```python
from build123d import *

# Parameters (mm, degrees)
SKETCH1_W           = 10.3
SKETCH1_H           = 5
BOSS_EXTRUDE1_DEPTH = 2.85
SKETCH2_W           = 5.7
SKETCH2_H           = 0.3
BOSS_EXTRUDE2_DEPTH = 5
SKETCH3_R           = 1.35
CUT_EXTRUDE1_DEPTH  = 5
SKETCH4_W           = 3
SKETCH4_H           = 3
BOSS_EXTRUDE3_DEPTH = 5
BOSS_EXTRUDE4_DEPTH = 0.15
LPATTERN1_COUNT     = 3
LPATTERN1_PITCH     = 3


with BuildPart() as part:
    # Sketch1 → Boss-Extrude1 (new body, symmetric)
    with BuildSketch(Plane.XY):
        Rectangle(SKETCH1_W, SKETCH1_H)
    extrude(amount=BOSS_EXTRUDE1_DEPTH, both=True)

    # Sketch2 → Boss-Extrude2 (add)
    with BuildSketch(Plane(origin=(5.15, 0, 0), x_dir=(0, 0, -1), z_dir=(1, 0, 0))):
        with Locations((0, 2.35)):
            Rectangle(SKETCH2_W, SKETCH2_H)
    boss_extrude2 = extrude(amount=BOSS_EXTRUDE2_DEPTH)

    # Sketch3 → Cut-Extrude1 (cut)
    with BuildSketch(Plane(origin=(0, 2.5, 0), x_dir=(1, 0, 0), z_dir=(0, 1, 0))):
        with Locations((7.65, 0)):
            Circle(SKETCH3_R)
    cut_extrude1 = extrude(amount=-CUT_EXTRUDE1_DEPTH, mode=Mode.SUBTRACT)

    # Mirror1: Boss-Extrude2, Cut-Extrude1 across plane
    add(boss_extrude2.mirror(Plane(origin=(0, 0, 0), x_dir=(0, 0, 1), z_dir=(1, 0, 0))))
    add(cut_extrude1.mirror(Plane(origin=(0, 0, 0), x_dir=(0, 0, 1), z_dir=(1, 0, 0))), mode=Mode.SUBTRACT)

    # Sketch4 → Boss-Extrude3 (add)
    with BuildSketch(Plane(origin=(0, 2.5, 0), x_dir=(1, 0, 0), z_dir=(0, 1, 0))):
        with Locations((2.65, 0)):
            Rectangle(SKETCH4_W, SKETCH4_H)
    extrude(amount=BOSS_EXTRUDE3_DEPTH)

    # Sketch5 → Boss-Extrude4 (add, symmetric)
    with BuildSketch(Plane.XY):
        with BuildLine():
            Line((-3.65, -2.5), (-2.15, -2.5))
            Line((-2.15, -2.5), (-2.15, -4.75))
            ThreePointArc((-2.15, -4.75), (-2.9, -5.5), (-3.65, -4.75))
            Line((-3.65, -4.75), (-3.65, -2.5))
        make_face()
        with BuildLine():
            Line((-2.45, -4.15), (-2.45, -4.75))
            ThreePointArc((-2.45, -4.75), (-2.9, -5.2), (-3.35, -4.75))
            Line((-3.35, -4.75), (-3.35, -4.15))
            ThreePointArc((-3.35, -4.15), (-2.9, -3.7), (-2.45, -4.15))
        make_face(mode=Mode.SUBTRACT)
    boss_extrude4 = extrude(amount=BOSS_EXTRUDE4_DEPTH, both=True)

    # LPattern1: Boss-Extrude4 ×3
    with Locations(*[(i * LPATTERN1_PITCH, 0, 0) for i in range(1, LPATTERN1_COUNT)]):
        add(boss_extrude4)


solid = part.part
```
Model file for the job. Use its own axes, mm. A direction names the side the tool comes from. Give positions to 0.01 mm unless a question says otherwise; leave off trailing zeros. Write each loop counter-clockwise with the first axis right and the second up, starting at its lowest first coordinate (ties: lowest second). Pieces come first, ordered by that corner, then holes. Notation, with made-up numbers: (-10.75, 83.25) -> (17.25, 83.25) arc R24 cw to (17.25, 121.25) -> close; hole circle Ø4 at (63.25, -12.5). An arc over 180 degrees is marked (long way). Use CSV: the item, a comma, the result in double quotes. Start each with the question number.
1) Pin check, flat tips, straight feed: P1, Ø3, axis at x = 7.65, z = 0, coming from the +Y side; P2, Ø0.8, axis at x = -2.5, y = -4, coming from the -Z side; P3, Ø1.5, axis at y = -4, z = -0.5, coming from the +X side. Stop position of each tip, or through.
2) Tool access for faces 1 (the flat face through (-3.2, -3.6, 0.15)), 2 (the flat face through (1.15, 5, 0)), 3 (the flat face through (2.8, -3.6, -0.15)), 4 (the flat face through (5.15, 0, 0)), 5 (the flat face through (-6, 2.2, 0)): list every direction of +Z, -Z, +X, -X, +Y, -Y with a clear straight run to the whole face (end or side of a thin tool).
3) Drill centre lines: L1, parallel to X at y = 2.45, z = 0; L2, parallel to Z at x = -7.65, y = 2.3; L3, parallel to Y at x = 1.25, z = -1.3. Where is each one in solid material? Low to high.
4) Cut at B-B on z = -1.75. List the corners of the cut face in (x, y), plus the area to 3 significant figures.
5) Cut at D-D on y = 4. List the corners of the cut face in (x, z), plus the area to 3 significant figures.
6) Cut at A-A on x = 3.1. List the corners of the cut face in (y, z).
7) Cut at C-C on x = -7.65. List the corners of the cut face in (y, z).
8) Two-plate mould, pull along X, no slides. Class faces 6 (the flat face through (-5.15, 0, 0)), 7 (the flat face through (-0.2, -3.6, 0.15)), 8 (the cylindrical face through (6.58, 2.35, 0.82)): released by +X, released by -X, zero draft, split by the parting line, or undercut.
Final values:
1,P1,"stops at y = 2.5"
1,P2,"stops at z = -0.15"
1,P3,"stops at x = 3.85"
2,face 1,"+Z, +X, -X, -Y"
2,face 2,"+Z, -Z, -X, +Y"
2,face 3,"-Z, +X, -X, -Y"
2,face 4,"+Z, -Z, +X, -Y"
2,face 5,"+Z, -Z, -X, -Y"
3,L1,"x = -10.15 to -9, -6.3 to 6.3, 9 to 10.15"
3,L2,"z = -2.85 to -1.35, 1.35 to 2.85"
3,L3,"y = -2.5 to 7.5"
4,outline,"(-10.15, 2.2) -> (-5.15, 2.2) -> (-5.15, -2.5) -> (5.15, -2.5) -> (5.15, 2.2) -> (10.15, 2.2) -> (10.15, 2.5) -> (-10.15, 2.5) -> close"
4,area,"54.5 mm2"
5,outline,"(1.15, -1.5) -> (4.15, -1.5) -> (4.15, 1.5) -> (1.15, 1.5) -> close"
5,area,"9.00 mm2"
6,outline,"(-5.5, -0.15) -> (-5.2, -0.15) -> (-5.2, 0.15) -> (-5.5, 0.15) -> close; (-3.7, -0.15) -> (-2.5, -0.15) -> (-2.5, -2.85) -> (2.5, -2.85) -> (2.5, -1.5) -> (7.5, -1.5) -> (7.5, 1.5) -> (2.5, 1.5) -> (2.5, 2.85) -> (-2.5, 2.85) -> (-2.5, 0.15) -> (-3.7, 0.15) -> close"
7,outline,"(2.2, -2.85) -> (2.5, -2.85) -> (2.5, -1.35) -> (2.2, -1.35) -> close; (2.2, 1.35) -> (2.5, 1.35) -> (2.5, 2.85) -> (2.2, 2.85) -> close"
8,face 6,"released by -X"
8,face 7,"zero draft"
8,face 8,"undercut"
